CAD build for the part. Positions are in the model's coordinates, mm. Give positions to 0.01 mm unless a question says otherwise; leave off trailing zeros. Write each loop counter-clockwise with the first axis right and the second up, starting at its lowest first coordinate (ties: lowest second). Pieces come first, ordered by that corner, then holes. Notation, with made-up numbers: (-6, -7) - (37, -7) arc R10 ccw to (37, 7) - close; hole circle Ø1 at (-7, 25). An arc over 180 degrees is marked (long way). Answer as a JSON object with one key per item and string values.
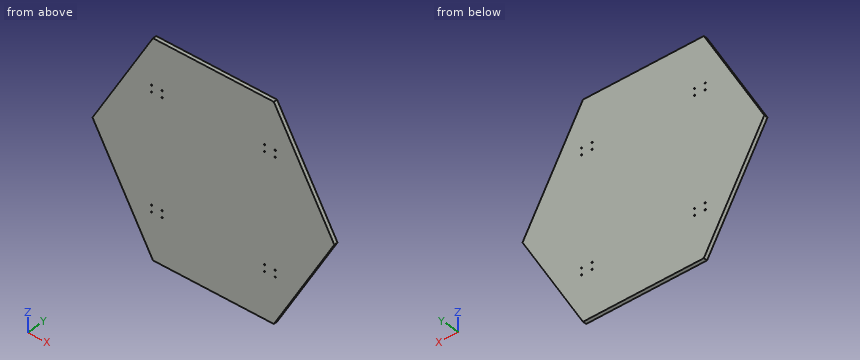
from build123d import *

# Parameters (mm, degrees)
BOSS_EXTRUDE1_DEPTH = 25.4
SKETCH5_R           = 4.191
CUT_EXTRUDE1_DEPTH  = 25.4


with BuildPart() as part:
    # Sketch1 → Boss-Extrude1 (new body)
    with BuildSketch(Plane(origin=(0, 0, 0), x_dir=(1, 0, 0), z_dir=(0, 1, 0))):
        Polygon((835.323484187, 0), (417.661742094, 723.411357684), (-417.661742094, 723.411357684), (-835.323484187, 0), (-417.661742094, -723.411357684), (417.661742094, -723.411357684), align=None)
    extrude(amount=BOSS_EXTRUDE1_DEPTH)

    # Sketch5 → Cut-Extrude1 (cut)
    with BuildSketch(Plane(origin=(0, 25.4, 0), x_dir=(1, 0, 0), z_dir=(0, 1, 0))):
        with Locations(Location((-353.949, 412.877, 0), (0, 0, 270))):
            Circle(SKETCH5_R)
        with Locations(Location((-427.101, 412.877, 0), (0, 0, 270))):
            Circle(SKETCH5_R)
        with Locations(Location((-427.101, 368.173, 0), (0, 0, 270))):
            Circle(SKETCH5_R)
        with Locations(Location((-353.949, 368.173, 0), (0, 0, 270))):
            Circle(SKETCH5_R)
        with Locations(Location((353.949, 368.173, 0), (0, 0, 270))):
            Circle(SKETCH5_R)
        with Locations(Location((427.101, 368.173, 0), (0, 0, 270))):
            Circle(SKETCH5_R)
        with Locations(Location((427.101, 412.877, 0), (0, 0, 270))):
            Circle(SKETCH5_R)
        with Locations(Location((353.949, 412.877, 0), (0, 0, 270))):
            Circle(SKETCH5_R)
        with Locations(Location((353.949, -412.877, 0), (0, 0, 270))):
            Circle(SKETCH5_R)
        with Locations(Location((427.101, -412.877, 0), (0, 0, 270))):
            Circle(SKETCH5_R)
        with Locations(Location((427.101, -368.173, 0), (0, 0, 270))):
            Circle(SKETCH5_R)
        with Locations(Location((353.949, -368.173, 0), (0, 0, 270))):
            Circle(SKETCH5_R)
        with Locations(Location((-353.949, -368.173, 0), (0, 0, 270))):
            Circle(SKETCH5_R)
        with Locations(Location((-427.101, -368.173, 0), (0, 0, 270))):
            Circle(SKETCH5_R)
        with Locations(Location((-427.101, -412.877, 0), (0, 0, 270))):
            Circle(SKETCH5_R)
        with Locations(Location((-353.949, -412.877, 0), (0, 0, 270))):
            Circle(SKETCH5_R)
    extrude(amount=-CUT_EXTRUDE1_DEPTH, mode=Mode.SUBTRACT)


solid = part.part
Item 1: Cut at A-A (y = 16). State how many separate pieces and enclosed holes the cut face has, and give its area (3 significant figures).
Entries:
{"separate pieces": "1", "enclosed holes": "16", "area": "1,810,000 mm2"}
Item 2: Probe line 1 (X direction, y = 10.5, z = -412); line 2 (X direction, y = 19.5, z = 356); line 3 (X direction, y = 10, z = 482). List the from-to ranges inside material, lowest first. Write a range as from..to.
Entries:
{"line 1": "-597.46..-431.2, -423..-358.05, -349.85..349.85, 358.05..423, 431.2..597.46", "line 2": "-629.79..629.79", "line 3": "-557.04..557.04"}
Item 3: Flat gauge pins, fed straight in: P1, Ø4, axis at y = 17.5, z = -18, coming from the +X side; P2, Ø5, axis at x = 427.101, z = 368.173, coming from the +Y side; P3, Ø11, axis at x = 353.949, z = 412.877, coming from the -Y side; P4, Ø1.5, axis at y = 17, z = -182.5, coming from the +X side. Where does each tip first touch, or does it go through?
Entries:
{"P1": "x = 826.09", "P2": "through", "P3": "y = 0", "P4": "x = 730.39"}
Item 4: Cut at C-C (x = 563). Give the cut face in (y, z).
Entries:
{"outline": "(0, -471.68) - (25.4, -471.68) - (25.4, 471.68) - (0, 471.68) - close"}
Item 5: Cut at B-B (z = -325). Give the cut face in (x, y).
Entries:
{"outline": "(-647.68, 0) - (647.68, 0) - (647.68, 25.4) - (-647.68, 25.4) - close"}
